Here's how the part is built. I have some questions about the finished solid (model axes, mm). Face numbers are marked on the shaded views. Round coordinates to 2 decimals unless told otherwise and drop trailing zeros. Write each loop counter-clockwise with the first axis right and the second up, starting at its lowest first coordinate (ties: lowest second). Pieces come first, ordered by that corner, then holes. Notation, with made-up numbers: (60.25, -26.75) - (73.25, -26.75) arc R20 cw to (73.25, -10.75) - close; hole circle Ø11 at (-3, 33). An arc over 180 degrees is marked (long way). One line per item, written item: value. Start each with the question number.
Item 1: Imagine slicing it at B-B, the plane x = -144.5. Please give me the cut outline in (y, z).
Item 2: For P1, Ø4.5, axis at x = 159, z = 10, coming from the -Y side; P2, Ø6, axis at x = 124, y = 129, coming from the -Z side; P3, Ø6, axis at x = -83, z = 3.5, coming from the +Y side; P4, Ø2, axis at x = 39.5, z = 11, coming from the +Y side, each with a flat end and sliding along its axis, tell me the tip position at first contact or that it passes through.
Item 3: If I drill on line 1 (X direction, y = 154, z = 5.75); line 2 (Y direction, x = -30, z = 5.5); line 3 (Y direction, x = -145.5, z = 7.25), over which ranges is the centre line in solid material (lowest first)?
Item 4: Imagine slicing it at A-A, the plane y = -11. Please give me the cut outline in (x, z), then the cut area to 3 significant figures.
Item 5: Imagine slicing it at C-C, the plane y = 177.5. Please give me the cut outline in (x, z).
Item 6: Thinking about a two-plate mould opening in Z: for the marked faces 1 and 2, which applies, released by +Z, released by -Z, zero draft, split by the parting line, or undercut?
Item 7: Imagine slicing it at D-D, the plane z = 8. Count the separate pieces of the cut face and the enclosed holes in it, then the cut area to 3 significant figures.
```python
from build123d import *

# Parameters (mm, degrees)
SKETCH1_W           = 30
SKETCH1_H           = 14.936006603
SKETCH1_H_2         = 15
BOSS_EXTRUDE1_DEPTH = 15


with BuildPart() as part:
    # Sketch1 → Boss-Extrude1 (new body)
    with BuildSketch(Plane.XY):
        with BuildLine():
            Line((169.965634662, 155), (169.965634662, 188))
            ThreePointArc((169.965634662, 188), (161.178838098, 209.213203436), (139.965634662, 218))
            Line((139.965634662, 218), (69.465634662, 218))
            ThreePointArc((69.465634662, 218), (55.323499038, 212.142135624), (49.465634662, 198))
            Line((49.465634662, 198), (49.465634662, 190))
            ThreePointArc((49.465634662, 190), (43.607770286, 175.857864376), (29.465634662, 170))
            Line((29.465634662, 170), (-49.534365338, 170))
            ThreePointArc((-49.534365338, 170), (-63.676500962, 175.857864376), (-69.534365338, 190))
            Line((-69.534365338, 190), (-69.534365338, 198))
            ThreePointArc((-69.534365338, 198), (-75.392229714, 212.142135624), (-89.534365338, 218))
            Line((-89.534365338, 218), (-160.034365338, 218))
            ThreePointArc((-160.034365338, 218), (-181.247568774, 209.213203436), (-190.034365338, 188))
            Line((-190.034365338, 188), (-190.034365338, -48))
            ThreePointArc((-190.034365338, -48), (-181.247568774, -69.213203436), (-160.034365338, -78))
            Line((-160.034365338, -78), (-89.534365338, -78))
            ThreePointArc((-89.534365338, -78), (-75.392229714, -72.142135624), (-69.534365338, -58))
            Line((-69.534365338, -58), (-69.534365338, -50))
            ThreePointArc((-69.534365338, -50), (-63.676500962, -35.857864376), (-49.534365338, -30))
            Line((-49.534365338, -30), (29.465634662, -30))
            ThreePointArc((29.465634662, -30), (43.607770286, -35.857864376), (49.465634662, -50))
            Line((49.465634662, -50), (49.465634662, -58))
            ThreePointArc((49.465634662, -58), (55.323499038, -72.142135624), (69.465634662, -78))
            Line((69.465634662, -78), (139.965634662, -78))
            ThreePointArc((139.965634662, -78), (161.178838098, -69.213203436), (169.965634662, -48))
            Line((169.965634662, -48), (169.965634662, -15))
            Line((169.965634662, -15), (140, -15))
            Line((140, -15), (140, 0))
            Line((140, 0), (169.965634662, 0))
            Line((169.965634662, 0), (169.965634662, 140))
            Line((169.965634662, 140), (140, 140))
            Line((140, 140), (140, 155))
            Line((140, 155), (169.965634662, 155))
        make_face()
        with Locations((-155, -7.497163522)):
            Rectangle(SKETCH1_W, SKETCH1_H, mode=Mode.SUBTRACT)
        with Locations((-95, -7.497163522)):
            Rectangle(SKETCH1_W, SKETCH1_H, mode=Mode.SUBTRACT)
        with Locations((-35, -7.497163522)):
            Rectangle(SKETCH1_W, SKETCH1_H, mode=Mode.SUBTRACT)
        with Locations((35, -7.5)):
            Rectangle(SKETCH1_W, SKETCH1_H_2, mode=Mode.SUBTRACT)
        with Locations((95, -7.5)):
            Rectangle(SKETCH1_W, SKETCH1_H_2, mode=Mode.SUBTRACT)
        with Locations((-155, 147.497163521)):
            Rectangle(SKETCH1_W, SKETCH1_H, mode=Mode.SUBTRACT)
        with Locations((-95, 147.497163521)):
            Rectangle(SKETCH1_W, SKETCH1_H, mode=Mode.SUBTRACT)
        with Locations((-35, 147.497163521)):
            Rectangle(SKETCH1_W, SKETCH1_H, mode=Mode.SUBTRACT)
        with Locations((35, 147.5)):
            Rectangle(SKETCH1_W, SKETCH1_H_2, mode=Mode.SUBTRACT)
        with Locations((95, 147.5)):
            Rectangle(SKETCH1_W, SKETCH1_H_2, mode=Mode.SUBTRACT)
    extrude(amount=BOSS_EXTRUDE1_DEPTH)


solid = part.part
```
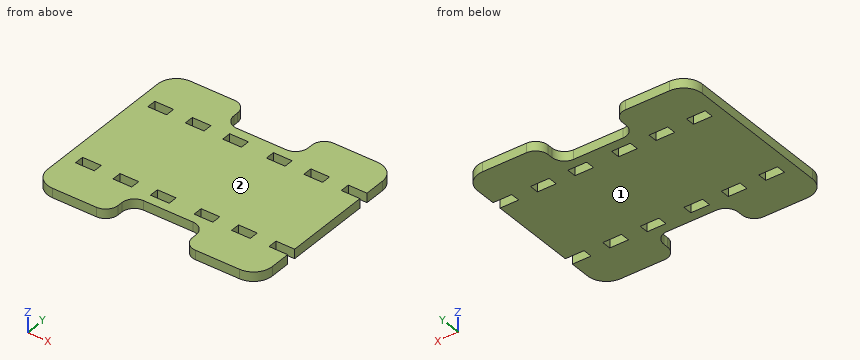
Values follow:
1. outline: (-78, 0) - (-14.97, 0) - (-14.97, 15) - (-78, 15) - close; (-0.03, 0) - (140.03, 0) - (140.03, 15) - (-0.03, 15) - close; (154.97, 0) - (218, 0) - (218, 15) - (154.97, 15) - close
2. P1: stops at y = -72.87
2. P2: stops at z = 0
2. P3: stops at y = 217.69
2. P4: stops at y = 173.32
3. line 1: x = -190.03 to -170, -140 to -110, -80 to -50, -20 to 20, 50 to 80, 110 to 140
3. line 2: y = -30 to -14.97, -0.03 to 140.03, 154.97 to 170
3. line 3: y = -78 to -14.97, -0.03 to 140.03, 154.97 to 218
4. outline: (-190.03, 0) - (-170, 0) - (-170, 15) - (-190.03, 15) - close; (-140, 0) - (-110, 0) - (-110, 15) - (-140, 15) - close; (-80, 0) - (-50, 0) - (-50, 15) - (-80, 15) - close; (-20, 0) - (20, 0) - (20, 15) - (-20, 15) - close; (50, 0) - (80, 0) - (80, 15) - (50, 15) - close; (110, 0) - (140, 0) - (140, 15) - (110, 15) - close
4. area: 2,700 mm^2
5. outline: (-190.03, 0) - (-65.15, 0) - (-65.15, 15) - (-190.03, 15) - close; (45.08, 0) - (169.97, 0) - (169.97, 15) - (45.08, 15) - close
6. face 1: released by -Z
6. face 2: released by +Z
7. separate pieces: 1
7. enclosed holes: 10
7. area: 89,000 mm^2
